from build123d import *

# Parameters (mm, degrees)
SKETCH1_W               = 57.3
SKETCH1_H               = 57.3
BOSS_EXTRUDE1_DEPTH     = 76.5
SKETCH2_W               = 9.55
SKETCH2_H               = 9.55
CUT_EXTRUDE1_DEPTH      = 72
MIRROR2_COPY_1_SKETCH_W = 9.55
MIRROR2_COPY_1_SKETCH_H = 9.55
MIRROR2_COPY_1_DEPTH    = 72
SKETCH3_R               = 19.1
BOSS_EXTRUDE2_DEPTH     = 1.6
SKETCH4_R               = 3
BOSS_EXTRUDE3_DEPTH     = 20.4
SKETCH5_R               = 2.7
CUT_EXTRUDE2_DEPTH      = 4.5
FILLET2_R               = 3
BOSS_EXTRUDE4_DEPTH     = 1.6
BOSS_EXTRUDE5_DEPTH     = 5.1
SKETCH9_R               = 3
CUT_EXTRUDE3_DEPTH      = 5.1


with BuildPart() as part:
    # Sketch1 → Boss-Extrude1 (new body)
    with BuildSketch(Plane(origin=(0, 0, 0), x_dir=(1, 0, 0), z_dir=(0, 1, 0))):
        Rectangle(SKETCH1_W, SKETCH1_H)
    extrude(amount=BOSS_EXTRUDE1_DEPTH)

    # Sketch2 → Cut-Extrude1 (cut)
    with BuildSketch(Plane.XZ):
        with Locations((-23.875, 23.875)):
            Rectangle(SKETCH2_W, SKETCH2_H)
    cut_extrude1 = extrude(amount=-CUT_EXTRUDE1_DEPTH, mode=Mode.SUBTRACT)

    # Mirror1: Cut-Extrude1 across plane
    add(cut_extrude1.mirror(Plane(origin=(0, 0, 0), x_dir=(0, 0, 1), z_dir=(1, 0, 0))), mode=Mode.SUBTRACT)

    # Mirror2: Cut-Extrude1 across plane
    add(cut_extrude1.mirror(Plane.XY), mode=Mode.SUBTRACT)

    # Mirror2 copy 1 sketch → Mirror2 copy 1 (cut)
    with BuildSketch(Plane(origin=(0, 0, 0), x_dir=(-1, 0, 0), z_dir=(0, -1, 0))):
        with Locations((-23.875, 23.875)):
            Rectangle(MIRROR2_COPY_1_SKETCH_W, MIRROR2_COPY_1_SKETCH_H)
    extrude(amount=-MIRROR2_COPY_1_DEPTH, mode=Mode.SUBTRACT)

    # Sketch3 → Boss-Extrude2 (add)
    with BuildSketch(Plane(origin=(0, 76.5, 0), x_dir=(1, 0, 0), z_dir=(0, 1, 0))):
        Circle(SKETCH3_R)
    extrude(amount=BOSS_EXTRUDE2_DEPTH)

    # Sketch4 → Boss-Extrude3 (add)
    with BuildSketch(Plane(origin=(0, 78.1, 0), x_dir=(1, 0, 0), z_dir=(0, 1, 0))):
        Circle(SKETCH4_R)
    extrude(amount=BOSS_EXTRUDE3_DEPTH)

    # Sketch5 → Cut-Extrude2 (cut)
    with BuildSketch(Plane(origin=(0, 76.5, 0), x_dir=(1, 0, 0), z_dir=(0, 1, 0))):
        with Locations((-23.55, 23.55)):
            Circle(SKETCH5_R)
        with Locations((23.55, 23.55)):
            Circle(SKETCH5_R)
        with Locations((23.55, -23.55)):
            Circle(SKETCH5_R)
        with Locations((-23.55, -23.55)):
            Circle(SKETCH5_R)
    extrude(amount=-CUT_EXTRUDE2_DEPTH, mode=Mode.SUBTRACT)

    # Fillet2
    fillet2_edges = [part.edges().sort_by_distance(p)[0] for p in [
        (-28.65, 74.25, -28.65),
        (28.65, 74.25, -28.65),
        (28.65, 74.25, 28.65),
        (-28.65, 74.25, 28.65),
    ]]
    fillet(fillet2_edges, radius=FILLET2_R)

    # Sketch6 → Boss-Extrude4 (add)
    with BuildSketch(Plane.ZY.offset(28.65)):
        Polygon((0, 0), (5.45, 0), (5.45, 9.6), (-5.45, 9.6), (-5.45, 0), align=None)
    extrude(amount=BOSS_EXTRUDE4_DEPTH)

    # Sketch7 → Boss-Extrude5 (add)
    with BuildSketch(Plane.ZY.offset(30.25)):
        Polygon((0, 0), (-4, 0), (-4, 2), (4, 2), (4, 0), align=None)
    extrude(amount=BOSS_EXTRUDE5_DEPTH)

    # Sketch9 → Cut-Extrude3 (cut)
    with BuildSketch(Plane.XZ):
        Circle(SKETCH9_R)
    extrude(amount=-CUT_EXTRUDE3_DEPTH, mode=Mode.SUBTRACT)


solid = part.part
Read the model definition and answer for the solid it produces. Units are mm, in the model's axes. A direction names the side the tool comes from. Round coordinates to 2 decimals unless told otherwise and drop trailing zeros. Write each loop counter-clockwise with the first axis right and the second up, starting at its lowest first coordinate (ties: lowest second). Pieces come first, ordered by that corner, then holes. Notation, with made-up numbers: (-2.75, 5) - (26.25, 5) arc R22 cw to (26.25, 20) - close; hole circle Ø5 at (-38.5, 52.25). An arc over 180 degrees is marked (long way). One line per question, with ' | ' between items. Start each with the question number.
1. Each of these flat-tipped pins is pushed along its axis until it touches: pin 1 (11.5 mm diameter, centred on x = -6.5, z = 5.5, fed in from +Y); pin 2 (4 mm diameter, centred on y = 35, z = 0, fed in from -X); pin 3 (8.5 mm diameter, centred on x = 23.55, z = 23.55, fed in from +Y); pin 4 (8 mm diameter, centred on x = -2, z = -19.5, fed in from +Y). Where does it stop, or does it pass through?
2. Section C-C (y = 19) is taken. Determine the outline of the cut face in (x, z), and give its area (3 significant figures).
3. For faces 1 (the face through (-33, 1, 4)), 2 (the face through (-26.1, 72, 25)), 3 (the face through (-33, 1, -4)), 4 (the face through (19.1, 35, 24)), 5 (the face through (-33, 2, 0)), determine the directions among +Z, -Z, +X, -X, +Y, -Y from which every point of the face is accessible in a straight line to the end or side of a thin tool.
4. Section D-D (z = 0) is taken. Determine the outline of the cut face in (x, y), and give its area (3 significant figures).
5. Section B-B (x = -23.55) is taken. Determine the outline of the cut face in (y, z).
6. Section A-A (z = 23.55) is taken. Determine the outline of the cut face in (x, y).
7. Find the intervals of material crossed by probe 1 along Z at (x, y) = (23.55, 73.4); probe 2 along Y at (x, z) = (-6.5, -16), in increasing order. Write a range as [from, to].
8. For a pull along Z with two mould halves and no side action, classify faces 6 (the face through (-28.65, 38, 0)), 7 (the face through (-24.135, 74.282, -20.914)), 8 (the face through (0, 38, 28.65)) as +Z half, -Z half, draft (parallel to the pull), parting line (faces both ways), or undercut.
Filled in:
1) pin 1: y = 98.5 | pin 2: x = -28.65 | pin 3: y = 76.5 | pin 4: y = 78.1
2) outline: (-28.65, -19.1) - (-19.1, -19.1) - (-19.1, -28.65) - (19.1, -28.65) - (19.1, -19.1) - (28.65, -19.1) - (28.65, 19.1) - (19.1, 19.1) - (19.1, 28.65) - (-19.1, 28.65) - (-19.1, 19.1) - (-28.65, 19.1) - close | area: 2,920 mm²
3) face 1: +Z, -X, +Y, -Y | face 2: +Z, -X, -Y | face 3: -Z, -X, +Y, -Y | face 4: +Z, +X, -Y | face 5: +Z, -Z, -X, +Y
4) outline: (-35.35, 0) - (-3, 0) - (-3, 5.1) - (3, 5.1) - (3, 0) - (28.65, 0) - (28.65, 76.5) - (19.1, 76.5) - (19.1, 78.1) - (3, 78.1) - (3, 98.5) - (-3, 98.5) - (-3, 78.1) - (-19.1, 78.1) - (-19.1, 76.5) - (-28.65, 76.5) - (-28.65, 9.6) - (-30.25, 9.6) - (-30.25, 2) - (-35.35, 2) - close | area: 4,560 mm²
5) outline: (0, -19.1) - (72, -19.1) - (72, -20.85) - (76.5, -20.85) - (76.5, 20.85) - (72, 20.85) - (72, 19.1) - (0, 19.1) - close; (72, -28.65) - (76.5, -28.65) - (76.5, -26.25) - (72, -26.25) - close; (72, 26.25) - (76.5, 26.25) - (76.5, 28.65) - (72, 28.65) - close
6) outline: (-28.65, 72) - (-26.25, 72) - (-26.25, 76.5) - (-28.65, 76.5) - close; (-20.85, 72) - (-19.1, 72) - (-19.1, 0) - (19.1, 0) - (19.1, 72) - (20.85, 72) - (20.85, 76.5) - (-20.85, 76.5) - close; (26.25, 72) - (28.65, 72) - (28.65, 76.5) - (26.25, 76.5) - close
7) probe 1: [-28.65, -26.25], [-20.85, 20.85], [26.25, 28.65] | probe 2: [0, 78.1]
8) face 6: draft | face 7: undercut | face 8: +Z half
